```python
from build123d import *

# Parameters (mm, degrees)
EXTRUDE_1_DEPTH     = 22.7
SKETCH_2_R          = 6.5
CUT_EXTRUDE_1_DEPTH = 33.480455662


with BuildPart() as part:
    # Эскиз1 → Бобышка-Вытянуть1 (new body)
    with BuildSketch(Plane.XY):
        with BuildLine():
            Line((-8.8, 0), (8.8, 0))
            Line((8.8, 0), (8.8, 17.9))
            ThreePointArc((8.8, 17.9), (0, 21.5), (-8.8, 17.9))
            Line((-8.8, 17.9), (-8.8, 0))
        make_face()
    extrude(amount=EXTRUDE_1_DEPTH)

    # Эскиз2 → Вырез-Вытянуть1 (cut, through all)
    with BuildSketch(Plane.XY.offset(22.7)):
        with Locations((0, 8.8)):
            Circle(SKETCH_2_R)
    extrude(amount=-CUT_EXTRUDE_1_DEPTH, mode=Mode.SUBTRACT)


solid = part.part
```
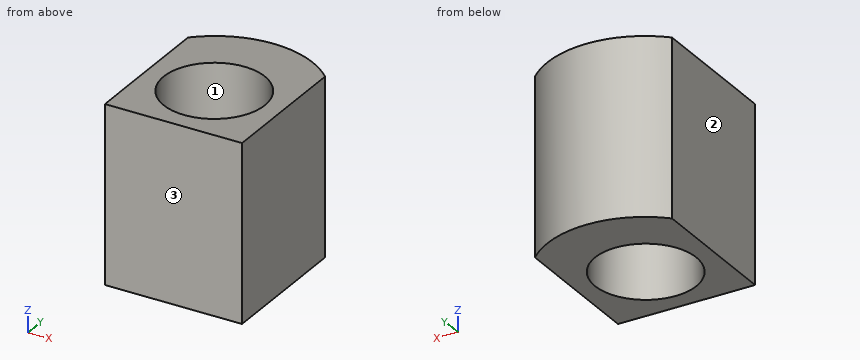
Model file for the job. Use its own axes, mm. Face numbers are marked on the shaded views. Give positions to 0.01 mm unless a question says otherwise; leave off trailing zeros. Write each loop counter-clockwise with the first axis right and the second up, starting at its lowest first coordinate (ties: lowest second). Pieces come first, ordered by that corner, then holes. Notation, with made-up numbers: (62.5, 36) - (120.5, 36) arc R32 ccw to (120.5, 66) - close; hole circle Ø10 at (-15.5, -31). An arc over 180 degrees is marked (long way). One line per question, with ' | ' between items. Start each with the question number.
(1) Wall check: line 1 along Y through (x, z) = (0, 8); line 2 along X through (y, z) = (8.75, 18.5); line 3 along X through (y, z) = (4.5, 13). Give the ranges that are in metal, low to high. Write a range as from..to.
(2) Two-plate mould, pull along Y, no slides. Class the marked faces 1, 2 and 3: +Y half, -Y half, draft (parallel to the pull), parting line (faces both ways), or undercut.
(3) Pin check, flat tips, straight feed: P1, Ø5, axis at x = 0, y = 11.5, coming from the +Z side; P2, Ø1.5, axis at x = 1.5, z = 13.5, coming from the +Y side. Stop position of each tip, or through.
(4) Slice it at B-B on x = 0. Write the cut outline in (y, z), plus the area to 3 significant figures.
(5) Slice it at A-A on y = 8.8. Write the cut outline in (x, z).
(6) Slice it at C-C on z = 8.25. Write the cut outline in (x, y), plus the area to 3 significant figures.
Results below:
1) line 1: 0..2.3, 15.3..21.5 | line 2: -8.8..-6.5, 6.5..8.8 | line 3: -8.8..-4.87, 4.87..8.8
2) face 1: undercut | face 2: draft | face 3: -Y half
3) P1: through | P2: y = 21.48
4) outline: (0, 0) - (2.3, 0) - (2.3, 22.7) - (0, 22.7) - close; (15.3, 0) - (21.5, 0) - (21.5, 22.7) - (15.3, 22.7) - close | area: 193 mm^2
5) outline: (-8.8, 0) - (-6.5, 0) - (-6.5, 22.7) - (-8.8, 22.7) - close; (6.5, 0) - (8.8, 0) - (8.8, 22.7) - (6.5, 22.7) - close
6) outline: (-8.8, 0) - (8.8, 0) - (8.8, 17.9) arc R12.56 ccw to (-8.8, 17.9) - close; hole circle Ø13 at (0, 8.8) | area: 226 mm^2
